```python
from build123d import *

# Parameters (mm, degrees)
SKETCH1_W            = 6.266
SKETCH1_H            = 19.6
SKETCH1_R            = 1.675
SKETCH1_W_2          = 52.832
SKETCH1_H_2          = 5
BOSS_EXTRUDE2_DEPTH  = 3.175
SKETCH3_W            = 30
SKETCH3_H            = 29.6
BOSS_EXTRUDE3_DEPTH  = 3.175
SKETCH4_R            = 4.75
CUT_EXTRUDE1_DEPTH   = 10
BOSS_EXTRUDE14_DEPTH = 3.175
CUT_EXTRUDE8_DEPTH   = 10
SKETCH24_R           = 1.675
CUT_EXTRUDE9_DEPTH   = 10
SKETCH25_R           = 3.675
SKETCH25_R_2         = 1.675
BOSS_EXTRUDE15_DEPTH = 3.175
SKETCH26_R           = 1.675
CUT_EXTRUDE12_DEPTH  = 3.175
SKETCH27_W           = 52.932563224
SKETCH27_H           = 23.005559857
BOSS_EXTRUDE16_DEPTH = 3.175
CUT_EXTRUDE14_DEPTH  = 10


with BuildPart() as part:
    # Sketch1 → Boss-Extrude2 (new body)
    # profile 1 of 4: a face of its own
    with BuildSketch(Plane.XY):
        with Locations((-23.283, 0)):
            Rectangle(SKETCH1_W, SKETCH1_H)
        with Locations((-23.95, -4.974)):
            Circle(SKETCH1_R, mode=Mode.SUBTRACT)
        with Locations((-23.95, 4.974)):
            Circle(SKETCH1_R, mode=Mode.SUBTRACT)
    # profile 2 of 4: a face of its own
    with BuildSketch(Plane.XY):
        with Locations((0, -12.3)):
            Rectangle(SKETCH1_W_2, SKETCH1_H_2)
    # profile 3 of 4: a face of its own
    with BuildSketch(Plane.XY):
        with Locations((0, 12.3)):
            Rectangle(SKETCH1_W_2, SKETCH1_H_2)
    # profile 4 of 4: a face of its own
    with BuildSketch(Plane.XY):
        with Locations((23.283, 0)):
            Rectangle(SKETCH1_W, SKETCH1_H)
        with Locations((23.95, -4.974)):
            Circle(SKETCH1_R, mode=Mode.SUBTRACT)
        with Locations((23.95, 4.974)):
            Circle(SKETCH1_R, mode=Mode.SUBTRACT)
    extrude(amount=BOSS_EXTRUDE2_DEPTH)

    # Sketch3 → Boss-Extrude3 (add)
    with BuildSketch(Plane.XY.offset(3.175)):
        with Locations((41.416, 0)):
            Rectangle(SKETCH3_W, SKETCH3_H)
    extrude(amount=-BOSS_EXTRUDE3_DEPTH)

    # Sketch4 → Cut-Extrude1 (cut)
    with BuildSketch(Plane(origin=(0, 0, 0), x_dir=(-1, 0, 0), z_dir=(0, 0, -1))):
        with Locations((-40.576, 7.77)):
            Circle(SKETCH4_R)
    extrude(amount=-CUT_EXTRUDE1_DEPTH, mode=Mode.SUBTRACT)

    # Sketch22 → Boss-Extrude14 (add)
    with BuildSketch(Plane(origin=(0, 0, 0), x_dir=(-1, 0, 0), z_dir=(0, 0, -1))):
        with BuildLine():
            ThreePointArc((-34.680262133, 14.8), (-40.576, 16.945), (-46.471737867, 14.8))
            Line((-46.471737867, 14.8), (-34.680262133, 14.8))
        make_face()
    extrude(amount=-BOSS_EXTRUDE14_DEPTH)

    # Sketch23 → Cut-Extrude8 (cut)
    with BuildSketch(Plane(origin=(0, 0, 0), x_dir=(-1, 0, 0), z_dir=(0, 0, -1))):
        with BuildLine():
            Line((-49.751, -14.8), (-49.751, 7.77))
            ThreePointArc((-49.751, 7.77), (-48.890866804, 11.648609936), (-46.471737867, 14.8))
            Line((-46.471737867, 14.8), (-56.416, 14.8))
            Line((-56.416, 14.8), (-56.416, -14.8))
            Line((-56.416, -14.8), (-49.751, -14.8))
        make_face()
    extrude(amount=-CUT_EXTRUDE8_DEPTH, mode=Mode.SUBTRACT)

    # Sketch24 → Cut-Extrude9 (cut)
    with BuildSketch(Plane(origin=(0, 0, 0), x_dir=(-1, 0, 0), z_dir=(0, 0, -1))):
        with Locations((23.736, 13.59)):
            Circle(SKETCH24_R)
    extrude(amount=-CUT_EXTRUDE9_DEPTH, mode=Mode.SUBTRACT)

    # Sketch25 → Boss-Extrude15 (add)
    # profile 1 of 3: a face of its own
    with BuildSketch(Plane(origin=(0, 0, 0), x_dir=(-1, 0, 0), z_dir=(0, 0, -1))):
        with Locations((23.95, -4.974)):
            Circle(SKETCH25_R)
        with Locations(Location((23.95, -4.974, 0), (0, 0, 180))):
            Circle(SKETCH25_R_2, mode=Mode.SUBTRACT)
    # profile 2 of 3: a face of its own
    with BuildSketch(Plane(origin=(0, 0, 0), x_dir=(-1, 0, 0), z_dir=(0, 0, -1))):
        with Locations((23.95, 4.974)):
            Circle(SKETCH25_R)
        with Locations(Location((23.95, 4.974, 0), (0, 0, 180))):
            Circle(SKETCH25_R_2, mode=Mode.SUBTRACT)
    # profile 3 of 3: a face of its own
    with BuildSketch(Plane(origin=(0, 0, 0), x_dir=(-1, 0, 0), z_dir=(0, 0, -1))):
        with Locations((23.736, 13.59)):
            Circle(SKETCH25_R)
        with Locations((23.736, 13.59)):
            Circle(SKETCH25_R_2, mode=Mode.SUBTRACT)
    extrude(amount=-BOSS_EXTRUDE15_DEPTH)

    # Sketch26 → Cut-Extrude12 (cut)
    with BuildSketch(Plane(origin=(0, 0, 0), x_dir=(-1, 0, 0), z_dir=(0, 0, -1))):
        with Locations((-46.076, -11.125)):
            Circle(SKETCH26_R)
    extrude(amount=-CUT_EXTRUDE12_DEPTH, mode=Mode.SUBTRACT)

    # Sketch27 → Boss-Extrude16 (add)
    with BuildSketch(Plane(origin=(0, 0, 0), x_dir=(-1, 0, 0), z_dir=(0, 0, -1))):
        with Locations((-0.417160697, -0.481381251)):
            Rectangle(SKETCH27_W, SKETCH27_H)
    extrude(amount=-BOSS_EXTRUDE16_DEPTH)

    # Sketch28 → Cut-Extrude14 (cut)
    with BuildSketch(Plane(origin=(0, 0, 0), x_dir=(-1, 0, 0), z_dir=(0, 0, -1))):
        Polygon((26.416, 8.97792488), (26.416, -8.885991227), (33.695668031, -3.414754928), align=None)
    extrude(amount=-CUT_EXTRUDE14_DEPTH, mode=Mode.SUBTRACT)


solid = part.part
```
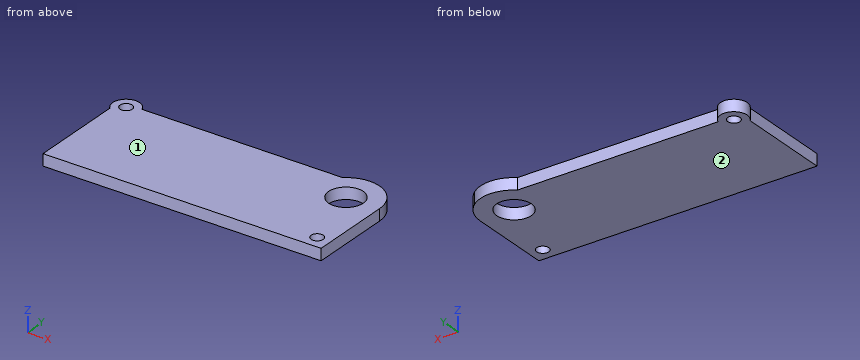
The listing builds one solid part. Answer for the finished solid, in the listing's coordinates (mm). Face numbers are marked on the shaded views. Coordinates: 2 decimals unless noted, no trailing zeros. Write each loop counter-clockwise with the first axis right and the second up, starting at its lowest first coordinate (ties: lowest second). Pieces come first, ordered by that corner, then holes. Notation, with made-up numbers: (-22.5, 77) -> (34.5, 77) arc R17 cw to (34.5, 110) -> close; hole circle Ø8 at (29, -39). An arc over 180 degrees is marked (long way). Write each question's results on one line, items separated by ' | '. Start each with the question number.
1) A cutting plane is placed at A-A (z = 1.1). Determine the outline of the cut face in (x, y) (3 decimals).
2) A cutting plane is placed at B-B (x = 38.5). Determine the outline of the cut face in (y, z) (3 decimals).
3) A cutting plane is placed at D-D (x = 30). Determine the outline of the cut face in (y, z) (3 decimals).
4) A cutting plane is placed at C-C (y = 6.5). Determine the outline of the cut face in (x, z) (3 decimals), then the cut area to 3 significant figures.
5) For a pull along Z with two mould halves and no side action, classify the marked faces 1 and 2 as +Z half, -Z half, draft (parallel to the pull), parting line (faces both ways), or undercut.
6) Straight lines are drawn through the part: probe 1 along X at (y, z) = (-6, 1.8); probe 2 along Y at (x, z) = (21, 2.7); probe 3 along Y at (x, z) = (43.5, 2.9). For each, find the intervals that lie inside material, in ascending order.
7) Flat-ended cylindrical pins translate along their axes: pin 1 Ø1 at (y, z) = (-1, 2) entering from -X; pin 2 Ø1 at (x, z) = (18, 2) entering from +Y; pin 3 Ø2.5 at (x, y) = (-23.736, 13.59) entering from -Z. Find the tip coordinate at first contact, or state that the pin passes through.
Values follow:
1) outline: (-26.416, -14.8) -> (49.751, -14.8) -> (49.751, 7.77) arc R9.175 ccw to (34.68, 14.8) -> (-20.266, 14.8) arc R3.675 ccw (long way) to (-26.416, 11.075) -> close; hole circle Ø3.35 at (-23.736, 13.59); hole circle Ø9.5 at (40.576, 7.77); hole circle Ø3.35 at (46.076, -11.125)
2) outline: (-14.8, 0) -> (3.498, 0) -> (3.498, 3.175) -> (-14.8, 3.175) -> close; (12.042, 0) -> (16.707, 0) -> (16.707, 3.175) -> (12.042, 3.175) -> close
3) outline: (-14.8, 0) -> (14.8, 0) -> (14.8, 3.175) -> (-14.8, 3.175) -> close
4) outline: (-26.416, 0) -> (35.999, 0) -> (35.999, 3.175) -> (-26.416, 3.175) -> close; (45.153, 0) -> (49.751, 0) -> (49.751, 3.175) -> (45.153, 3.175) -> close | area: 213 mm²
5) face 1: +Z half | face 2: -Z half
6) probe 1: -26.42 to 49.75 | probe 2: -14.8 to 14.8 | probe 3: -14.8 to 4.03, 11.51 to 16.47
7) pin 1: x = -26.42 | pin 2: y = 14.8 | pin 3: through
